Work out the finished part from the listing and answer in its coordinate system (mm). Face numbers are marked on the shaded views. A direction names the side the tool comes from. Coordinates: 2 decimals unless noted, no trailing zeros. Write each loop counter-clockwise with the first axis right and the second up, starting at its lowest first coordinate (ties: lowest second). Pieces come first, ordered by that corner, then holes. Notation, with made-up numbers: (62.5, 40) - (76.5, 40) arc R37 ccw to (76.5, 79) - close; hole circle Ø10 at (28.25, 61.25). An arc over 180 degrees is marked (long way). Use CSV: the item, a comma, the result in double quotes. Start each with the question number.
from build123d import *

# Parameters (mm, degrees)
BOSS_EXTRUDE1_DEPTH = 9.2
CUT_EXTRUDE3_DEPTH  = 50.582658259
SKETCH18_R          = 2.25
CUT_EXTRUDE10_DEPTH = 10
BOSS_EXTRUDE3_DEPTH = 2.1
FILLET3_R           = 1
CUT_EXTRUDE8_DEPTH  = 51.04637849
SKETCH13_R          = 0.25
SKETCH17_R          = 3.085
CUT_EXTRUDE9_DEPTH  = 8.2
CHAMFER1_SIZE       = 1


with BuildPart() as part:
    # Sketch1 → Boss-Extrude1 (new body)
    with BuildSketch(Plane(origin=(0, 0, 0), x_dir=(1, 0, 0), z_dir=(0, 1, 0))):
        with BuildLine():
            Line((-17, -44), (17, -44))
            ThreePointArc((17, -44), (20.535533906, -42.535533906), (22, -39))
            Line((22, -39), (22, 39))
            ThreePointArc((22, 39), (20.535533906, 42.535533906), (17, 44))
            Line((17, 44), (-17, 44))
            ThreePointArc((-17, 44), (-20.535533906, 42.535533906), (-22, 39))
            Line((-22, 39), (-22, -39))
            ThreePointArc((-22, -39), (-20.535533906, -42.535533906), (-17, -44))
        make_face()
    extrude(amount=BOSS_EXTRUDE1_DEPTH)

    # Sketch4 → Cut-Extrude3 (cut, through all)
    with BuildSketch(Plane(origin=(0, 6.2, 0), x_dir=(-1, 0, 0), z_dir=(0, -1, 0))):
        with BuildLine():
            Line((-16, -32), (-16, 32))
            ThreePointArc((-16, 32), (-15.121320344, 34.121320344), (-13, 35))
            Line((-13, 35), (13, 35))
            ThreePointArc((13, 35), (15.121320344, 34.121320344), (16, 32))
            Line((16, 32), (16, -32))
            ThreePointArc((16, -32), (15.121320344, -34.121320344), (13, -35))
            Line((13, -35), (-13, -35))
            ThreePointArc((-13, -35), (-15.121320344, -34.121320344), (-16, -32))
        make_face()
    extrude(amount=CUT_EXTRUDE3_DEPTH, mode=Mode.SUBTRACT)

    # Sketch18 → Cut-Extrude10 (cut)
    with BuildSketch(Plane.XZ.offset(-6.2)):
        with Locations(Location((-12, 25, 0), (0, 0, 270))):
            Circle(SKETCH18_R)
        with BuildLine():
            Line((-3, -33), (3, -33))
            ThreePointArc((3, -33), (4.414213562, -32.414213562), (5, -31))
            Line((5, -31), (5, 31))
            ThreePointArc((5, 31), (4.414213562, 32.414213562), (3, 33))
            Line((3, 33), (-3, 33))
            ThreePointArc((-3, 33), (-4.414213562, 32.414213562), (-5, 31))
            Line((-5, 31), (-5, -31))
            ThreePointArc((-5, -31), (-4.414213562, -32.414213562), (-3, -33))
        make_face()
    extrude(amount=-CUT_EXTRUDE10_DEPTH, mode=Mode.SUBTRACT)

    # Sketch9 → Boss-Extrude3 (add)
    with BuildSketch(Plane(origin=(0, 9.2, 0), x_dir=(1, 0, 0), z_dir=(0, 1, 0))):
        with BuildLine():
            Line((-17, -44), (17, -44))
            ThreePointArc((17, -44), (20.535533906, -42.535533906), (22, -39))
            Line((22, -39), (22, 39))
            ThreePointArc((22, 39), (20.535533906, 42.535533906), (17, 44))
            Line((17, 44), (-17, 44))
            ThreePointArc((-17, 44), (-20.535533906, 42.535533906), (-22, 39))
            Line((-22, 39), (-22, -39))
            ThreePointArc((-22, -39), (-20.535533906, -42.535533906), (-17, -44))
        make_face()
        with BuildLine():
            Line((-17, -42), (17, -42))
            ThreePointArc((17, -42), (19.121320344, -41.121320344), (20, -39))
            Line((20, -39), (20, 39))
            ThreePointArc((20, 39), (19.121320344, 41.121320344), (17, 42))
            Line((17, 42), (-17, 42))
            ThreePointArc((-17, 42), (-19.121320344, 41.121320344), (-20, 39))
            Line((-20, 39), (-20, -39))
            ThreePointArc((-20, -39), (-19.121320344, -41.121320344), (-17, -42))
        make_face(mode=Mode.SUBTRACT)
    extrude(amount=BOSS_EXTRUDE3_DEPTH)

    # Fillet3
    fillet3_edges = [part.edges().sort_by_distance(p)[0] for p in [
        (22, 11.3, 0),
        (20.535533906, 11.3, -42.535533906),
        (0, 11.3, -44),
        (-20.535533906, 11.3, -42.535533906),
        (-22, 11.3, 0),
        (-20.535533906, 11.3, 42.535533906),
        (0, 11.3, 44),
        (20.535533906, 11.3, 42.535533906),
    ]]
    fillet(fillet3_edges, radius=FILLET3_R)

    # Sketch12 → Cut-Extrude8 (cut, through all)
    with BuildSketch(Plane(origin=(0, 9.2, 0), x_dir=(1, 0, 0), z_dir=(0, 1, 0))):
        with BuildLine():
            Line((-20.1, 39), (-20.1, -39))
            ThreePointArc((-20.1, -39), (-19.192031022, -41.192031022), (-17, -42.1))
            Line((-17, -42.1), (17, -42.1))
            ThreePointArc((17, -42.1), (19.192031022, -41.192031022), (20.1, -39))
            Line((20.1, -39), (20.1, 39))
            ThreePointArc((20.1, 39), (19.192031022, 41.192031022), (17, 42.1))
            Line((17, 42.1), (-17, 42.1))
            ThreePointArc((-17, 42.1), (-19.192031022, 41.192031022), (-20.1, 39))
        make_face()
        with BuildLine():
            Line((-20, 39), (-20, -39))
            ThreePointArc((-20, -39), (-19.121320344, -41.121320344), (-17, -42))
            Line((-17, -42), (17, -42))
            ThreePointArc((17, -42), (19.121320344, -41.121320344), (20, -39))
            Line((20, -39), (20, 39))
            ThreePointArc((20, 39), (19.121320344, 41.121320344), (17, 42))
            Line((17, 42), (-17, 42))
            ThreePointArc((-17, 42), (-19.121320344, 41.121320344), (-20, 39))
        make_face(mode=Mode.SUBTRACT)
    extrude(amount=CUT_EXTRUDE8_DEPTH, mode=Mode.SUBTRACT)

    # Cut-Sweep1: sweep along a path in Sketch14
    with BuildLine(Plane(origin=(0, 9.2, 0), x_dir=(1, 0, 0), z_dir=(0, 1, 0))) as cut_sweep1_path:
        Line((-20.1, 39), (-20.1, -39))
        ThreePointArc((-20.1, -39), (-19.192031022, -41.192031022), (-17, -42.1))
        Line((-17, -42.1), (17, -42.1))
        ThreePointArc((17, -42.1), (19.192031022, -41.192031022), (20.1, -39))
        Line((20.1, -39), (20.1, 39))
        ThreePointArc((20.1, 39), (19.192031022, 41.192031022), (17, 42.1))
        Line((17, 42.1), (-17, 42.1))
        ThreePointArc((-17, 42.1), (-19.192031022, 41.192031022), (-20.1, 39))
    # Sketch13 → Cut-Sweep1 (sweep, cut)
    with BuildSketch(Plane(origin=(0, 0, 0), x_dir=(0, 0, -1), z_dir=(1, 0, 0))):
        with Locations((41.958578644, 9.341421356)):
            Circle(SKETCH13_R)
    sweep(path=cut_sweep1_path.line, mode=Mode.SUBTRACT)

    # Sketch17 → Cut-Extrude9 (cut)
    with BuildSketch(Plane.XZ):
        with Locations(Location((-16, 38, 0), (0, 0, 270))):
            Circle(SKETCH17_R)
        with Locations(Location((16, 38, 0), (0, 0, 270))):
            Circle(SKETCH17_R)
        with Locations(Location((16, -38, 0), (0, 0, 270))):
            Circle(SKETCH17_R)
        with Locations(Location((-16, -38, 0), (0, 0, 270))):
            Circle(SKETCH17_R)
    extrude(amount=-CUT_EXTRUDE9_DEPTH, mode=Mode.SUBTRACT)

    # Chamfer1
    chamfer1_edges = [part.edges().sort_by_distance(p)[0] for p in [
        (22, 0, 0),
        (20.535533906, 0, 42.535533906),
        (0, 0, 44),
        (-20.535533906, 0, 42.535533906),
        (-22, 0, 0),
        (-20.535533906, 0, -42.535533906),
        (0, 0, -44),
        (20.535533906, 0, -42.535533906),
    ]]
    chamfer(chamfer1_edges, length=CHAMFER1_SIZE)


solid = part.part
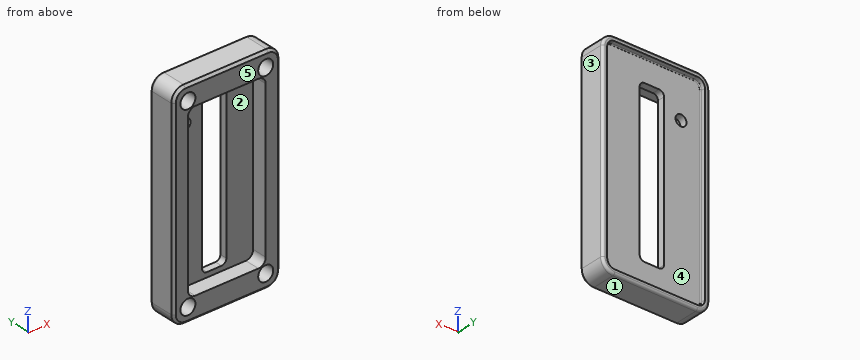
Item 1: A cutting plane is placed at A-A (x = -12). Determine the outline of the cut face in (y, z), then the cut area to 3 significant figures.
Item 2: Straight lines are drawn through the part: probe 1 along X at (y, z) = (5, -38) (3 decimals); probe 2 along X at (y, z) = (10, -28); probe 3 along X at (y, z) = (1.5, -11). For each, find the intervals that lie inside material, in ascending order. Write a range as [from, to].
Item 3: A cutting plane is placed at C-C (z = -19). Determine the outline of the cut face in (x, y).
Item 4: Determine the mould class of the marked faces 1, 2 and 3 for opening direction X: +X half, -X half, draft (parallel to the pull), parting line (faces both ways), or undercut.
Item 5: Each of these flat-tipped pins is pushed along its axis until it touches: pin 1 (1.5 mm diameter, centred on x = -7.5, z = 18.5, fed in from +Y); pin 2 (6 mm diameter, centred on x = -12, z = 25, fed in from -Y). Where does it stop, or does it pass through?
Item 6: A cutting plane is placed at B-B (y = 7). Determine the outline of the cut face in (x, z) (3 decimals), then the cut area to 3 significant figures.
Item 7: A cutting plane is placed at D-D (x = -7). Determine the outline of the cut face in (y, z).
Item 8: Which of the six approach directions +Z, -Z, +X, -X, +Y, -Y give full straight-line access (tool end or side, diameter ignored) to the marked faces 4 and 5?
Calculated:
1,outline,"(0, -43) - (1, -44) - (10.3, -44) arc R1 ccw to (11.3, -43) - (11.3, -42.1) - (9.55, -42.1) arc R0.25 cw (long way) to (9.2, -41.75) - (9.2, 22.75) - (6.2, 22.75) - (6.2, -35) - (0, -35) - close; (0, 35) - (6.2, 35) - (6.2, 27.25) - (9.2, 27.25) - (9.2, 41.75) arc R0.25 cw (long way) to (9.55, 42.1) - (11.3, 42.1) - (11.3, 43) arc R1 ccw to (10.3, 44) - (1, 44) - (0, 43) - close"
1,area,"369 mm²"
2,probe 1,"x = [-22, -19.085], [-12.915, 12.915], [19.085, 22]"
2,probe 2,"x = [-22, -20.1], [20.1, 22]"
2,probe 3,"x = [-22, -16], [16, 22]"
3,outline,"(-22, 1) - (-21, 0) - (-16, 0) - (-16, 6.2) - (-5, 6.2) - (-5, 9.2) - (-19.75, 9.2) arc R0.25 cw (long way) to (-20.1, 9.55) - (-20.1, 11.3) - (-21, 11.3) arc R1 ccw to (-22, 10.3) - close; (5, 6.2) - (16, 6.2) - (16, 0) - (21, 0) - (22, 1) - (22, 10.3) arc R1 ccw to (21, 11.3) - (20.1, 11.3) - (20.1, 9.55) arc R0.25 cw (long way) to (19.75, 9.2) - (5, 9.2) - close"
4,face 1,"draft"
4,face 2,"undercut"
4,face 3,"+X half"
5,pin 1,"stops at y = 9.2"
5,pin 2,"stops at y = 6.2"
6,outline,"(-22, -39) arc R5 ccw to (-17, -44) - (17, -44) arc R5 ccw to (22, -39) - (22, 39) arc R5 ccw to (17, 44) - (-17, 44) arc R5 ccw to (-22, 39) - close; hole circle Ø6.17 at (-16, -38); hole circle Ø6.17 at (-16, 38); hole circle Ø4.5 at (-12, 25); hole (-5, -31) arc R2 ccw to (-3, -33) - (3, -33) arc R2 ccw to (5, -31) - (5, 31) arc R2 ccw to (3, 33) - (-3, 33) arc R2 ccw to (-5, 31) - close; hole circle Ø6.17 at (16, -38); hole circle Ø6.17 at (16, 38)"
6,area,"3,060 mm²"
7,outline,"(0, -43) - (1, -44) - (10.3, -44) arc R1 ccw to (11.3, -43) - (11.3, -42.1) - (9.55, -42.1) arc R0.25 cw (long way) to (9.2, -41.75) - (9.2, 41.75) arc R0.25 cw (long way) to (9.55, 42.1) - (11.3, 42.1) - (11.3, 43) arc R1 ccw to (10.3, 44) - (1, 44) - (0, 43) - (0, 35) - (6.2, 35) - (6.2, -35) - (0, -35) - close"
8,face 4,"+Y"
8,face 5,"+Z, -Z, +X, -X, -Y"
